Input: dimensioned drawing with shaded views. Units: mm. Origin: part minimum x, y, z. Round coordinates to 2 decimals unless told otherwise and drop trailing zeros. Loops run counter-clockwise (first coordinate to the right, second up) from the corner with the lowest first, then second, coordinate; pieces in that order, holes last. Notation, with made-up numbers: M -29,-22.5 L 15,-22.5 A30 cw 15,5.5 Z; hole C 80.5,27 d6. An arc over 180 degrees is marked long. Return JSON: item names as keys, results as strings.
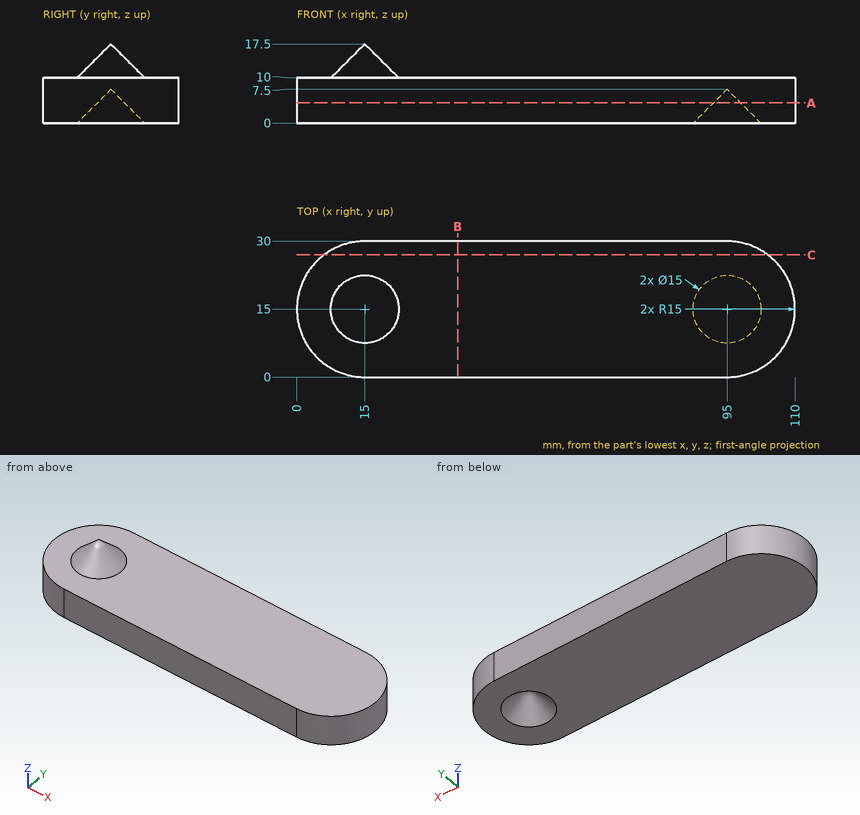
Q1. Section query B-B (x = 35.5). Output: boundary loops of the cut face in (y, z), plus the area to 3 significant figures.
Determined:
{"outline": "M 0,0 L 30,0 L 30,10 L 0,10 Z", "area": "300 mm^2"}
Q2. Section query A-A (z = 4.5). Output: boundary loops of the cut face in (x, y), plus the area to 3 significant figures.
Determined:
{"outline": "M 15,0 L 95,0 A15 ccw 95,30 L 15,30 A15 ccw Z; hole C 95,15 d6", "area": "3,080 mm^2"}
Q3. Material intervals for L1, parallel to Z at x = 26.5, y = 19; L2, parallel to X at y = 15.75, z = 4.25; L3, parallel to X at y = 10.25, z = 8.5, sorted ascending.
Determined:
{"L1": "z = 0 to 10", "L2": "x = 0.02 to 91.84, 98.16 to 109.98", "L3": "x = 0.77 to 109.23"}
Q4. Pin query (flat end, axial travel): pin 1 (1.5 mm diameter, centred on y = 6.5, z = 11.5, fed in from +X); pin 2 (8 mm diameter, centred on y = 14.5, z = 15.5, fed in from +X); pin 3 (9 mm diameter, centred on x = 49.5, y = 14, fed in from +Z). Return the tip coordinate at first contact, or that it passes through.
Determined:
{"pin 1": "passes through", "pin 2": "stops at x = 20.99", "pin 3": "stops at z = 10"}
Q5. Section query C-C (y = 27). Output: boundary loops of the cut face in (x, z), plus the area to 3 significant figures.
Determined:
{"outline": "M 6,0 L 104,0 L 104,10 L 6,10 Z", "area": "980 mm^2"}
